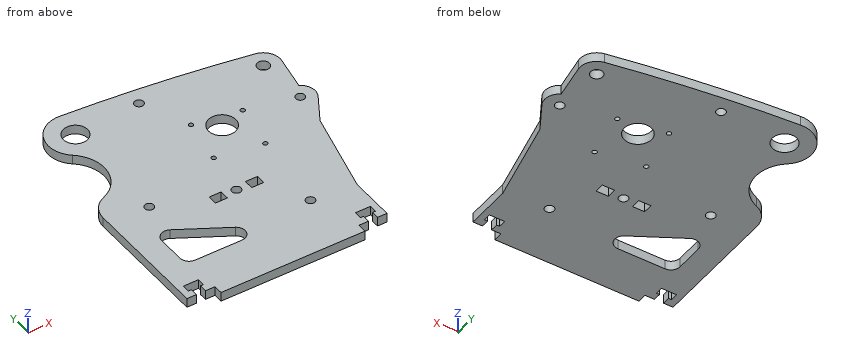
from build123d import *

# Parameters (mm, degrees)
SKETCH1_R           = 4
SKETCH1_R_2         = 8
SKETCH1_R_3         = 3
SKETCH1_R_4         = 9
BOSS_EXTRUDE1_DEPTH = 6.2
CUT_EXTRUDE1_REACH  = 156.506
SKETCH2_R           = 1.5
CUT_EXTRUDE2_REACH  = 156.506
CUT_EXTRUDE3_REACH  = 156.506
SKETCH4_R           = 3
SKETCH4_W           = 8
SKETCH4_H           = 6.2


with BuildPart() as part:
    # Sketch1 → Boss-Extrude1 (new body)
    with BuildSketch(Plane.XY):
        with BuildLine():
            Line((33.65, -83.5), (47, -26.5))
            Line((47, -26.5), (57.678304402, -8.5))
            ThreePointArc((57.678304402, -8.5), (58.708572703, -0.936463864), (54, 5.071686829))
            Line((54, 5.071686829), (58, 28.071686829))
            ThreePointArc((58, 28.071686829), (56.207110337, 36.277710094), (49.152329455, 40.836584722))
            ThreePointArc((49.152329455, 40.836584722), (-10.365453902, 50.052003716), (-70.318491494, 55.789927265))
            ThreePointArc((-70.318491494, 55.789927265), (-88.125314746, 44.440216148), (-82.611172846, 24.056567409))
            ThreePointArc((-82.611172846, 24.056567409), (-74.166284142, 2.579562371), (-88.533690885, -15.480213766))
            ThreePointArc((-88.533690885, -15.480213766), (-95.663024793, -21.178356395), (-98.35, -29.900534772))
            Line((-98.35, -29.900534772), (-98.35, -113))
            Line((-98.35, -113), (-79.85, -113))
            Line((-79.85, -113), (-79.85, -119))
            Line((-79.85, -119), (15.15, -119))
            Line((15.15, -119), (15.15, -113))
            Line((15.15, -113), (33.65, -113))
            Line((33.65, -113), (33.65, -83.5))
        make_face()
        with Locations(Location((47.15, 30, 0), (0, 0, 180))):
            Circle(SKETCH1_R, mode=Mode.SUBTRACT)
        with Locations(Location((-71.5, 38, 0), (0, 0, 180))):
            Circle(SKETCH1_R_2, mode=Mode.SUBTRACT)
        with Locations(Location((-27.65, 40.9, 0), (0, 0, 180))):
            Circle(SKETCH1_R_3, mode=Mode.SUBTRACT)
        with Locations(Location((4.85, -80.4, 0), (0, 0, 180))):
            Circle(SKETCH1_R_3, mode=Mode.SUBTRACT)
        with Locations(Location((49.25, -3.5, 0), (0, 0, 180))):
            Circle(SKETCH1_R_3, mode=Mode.SUBTRACT)
        with Locations(Location((-72, -36, 0), (0, 0, 180))):
            Circle(SKETCH1_R_3, mode=Mode.SUBTRACT)
        with Locations(Location((0, 0, 0), (0, 0, 180))):
            Circle(SKETCH1_R_4, mode=Mode.SUBTRACT)
        with BuildLine():
            Line((-82.35, -64), (-82.35, -82))
            ThreePointArc((-82.35, -82), (-80.592640687, -86.242640687), (-76.35, -88))
            Line((-76.35, -88), (-45.35, -88))
            ThreePointArc((-45.35, -88), (-39.556365472, -83.560063768), (-42.337186896, -76.81126632))
            Line((-42.337186896, -76.81126632), (-73.337186896, -58.81126632))
            ThreePointArc((-73.337186896, -58.81126632), (-79.343586593, -58.800150068), (-82.35, -64))
        make_face(mode=Mode.SUBTRACT)
    extrude(amount=BOSS_EXTRUDE1_DEPTH)

    # Sketch2 → Cut-Extrude1 (cut, up to next)
    with BuildSketch(Plane.XY.offset(6.2), mode=Mode.PRIVATE) as cut_extrude1_sk1:
        with Locations((-19.348702159, -20.792251556)):
            Circle(SKETCH2_R)
    cut_extrude1_tool1 = extrude(cut_extrude1_sk1.sketch, amount=-CUT_EXTRUDE1_REACH, mode=Mode.PRIVATE) & part.part
    # Sketch2 → Cut-Extrude1 (cut, up to next)
    with BuildSketch(Plane.XY.offset(6.2), mode=Mode.PRIVATE) as cut_extrude1_sk2:
        with Locations((11.192862241, -26.103827973)):
            Circle(SKETCH2_R)
    cut_extrude1_tool2 = extrude(cut_extrude1_sk2.sketch, amount=-CUT_EXTRUDE1_REACH, mode=Mode.PRIVATE) & part.part
    # Sketch2 → Cut-Extrude1 (cut, up to next)
    with BuildSketch(Plane.XY.offset(6.2), mode=Mode.PRIVATE) as cut_extrude1_sk3:
        with Locations((-14.037125741, 9.749312843)):
            Circle(SKETCH2_R)
    cut_extrude1_tool3 = extrude(cut_extrude1_sk3.sketch, amount=-CUT_EXTRUDE1_REACH, mode=Mode.PRIVATE) & part.part
    # Sketch2 → Cut-Extrude1 (cut, up to next)
    with BuildSketch(Plane.XY.offset(6.2), mode=Mode.PRIVATE) as cut_extrude1_sk4:
        with Locations((16.504438658, 4.437736426)):
            Circle(SKETCH2_R)
    cut_extrude1_tool4 = extrude(cut_extrude1_sk4.sketch, amount=-CUT_EXTRUDE1_REACH, mode=Mode.PRIVATE) & part.part
    add(cut_extrude1_tool1.solids().sort_by_distance((-19.348702, -20.792252, 6.2))[0], mode=Mode.SUBTRACT)
    add(cut_extrude1_tool2.solids().sort_by_distance((11.192862, -26.103828, 6.2))[0], mode=Mode.SUBTRACT)
    add(cut_extrude1_tool3.solids().sort_by_distance((-14.037126, 9.749313, 6.2))[0], mode=Mode.SUBTRACT)
    add(cut_extrude1_tool4.solids().sort_by_distance((16.504439, 4.437736, 6.2))[0], mode=Mode.SUBTRACT)

    # Sketch3 → Cut-Extrude2 (cut, up to next)
    with BuildSketch(Plane(origin=(0, 0, 0), x_dir=(-1, 0, 0), z_dir=(0, 0, -1)), mode=Mode.PRIVATE) as cut_extrude2_sk1:
        Polygon((-29.4, -103), (-19.4, -103), (-19.4, -108), (-21.4, -108), (-21.4, -113), (-27.4, -113), (-27.4, -108), (-29.4, -108), align=None)
    cut_extrude2_tool1 = extrude(cut_extrude2_sk1.sketch, amount=-CUT_EXTRUDE2_REACH, mode=Mode.PRIVATE) & part.part
    # Sketch3 → Cut-Extrude2 (cut, up to next)
    with BuildSketch(Plane(origin=(0, 0, 0), x_dir=(-1, 0, 0), z_dir=(0, 0, -1)), mode=Mode.PRIVATE) as cut_extrude2_sk2:
        Polygon((92.1, -113), (86.1, -113), (86.1, -108), (84.1, -108), (84.1, -103), (94.1, -103), (94.1, -108), (92.1, -108), align=None)
    cut_extrude2_tool2 = extrude(cut_extrude2_sk2.sketch, amount=-CUT_EXTRUDE2_REACH, mode=Mode.PRIVATE) & part.part
    add(cut_extrude2_tool1.solids().sort_by_distance((24.4, -107.375, 0))[0], mode=Mode.SUBTRACT)
    add(cut_extrude2_tool2.solids().sort_by_distance((-89.1, -107.375, 0))[0], mode=Mode.SUBTRACT)

    # Sketch4 → Cut-Extrude3 (cut, up to next)
    with BuildSketch(Plane.XY.offset(6.2), mode=Mode.PRIVATE) as cut_extrude3_sk1:
        with Locations((-24.05, -50.4)):
            Circle(SKETCH4_R)
    cut_extrude3_tool1 = extrude(cut_extrude3_sk1.sketch, amount=-CUT_EXTRUDE3_REACH, mode=Mode.PRIVATE) & part.part
    # Sketch4 → Cut-Extrude3 (cut, up to next)
    with BuildSketch(Plane.XY.offset(6.2), mode=Mode.PRIVATE) as cut_extrude3_sk2:
        with Locations((-36.05, -50.4)):
            Rectangle(SKETCH4_W, SKETCH4_H)
    cut_extrude3_tool2 = extrude(cut_extrude3_sk2.sketch, amount=-CUT_EXTRUDE3_REACH, mode=Mode.PRIVATE) & part.part
    # Sketch4 → Cut-Extrude3 (cut, up to next)
    with BuildSketch(Plane.XY.offset(6.2), mode=Mode.PRIVATE) as cut_extrude3_sk3:
        with Locations((-12.05, -50.4)):
            Rectangle(SKETCH4_W, SKETCH4_H)
    cut_extrude3_tool3 = extrude(cut_extrude3_sk3.sketch, amount=-CUT_EXTRUDE3_REACH, mode=Mode.PRIVATE) & part.part
    add(cut_extrude3_tool1.solids().sort_by_distance((-24.05, -50.4, 6.2))[0], mode=Mode.SUBTRACT)
    add(cut_extrude3_tool2.solids().sort_by_distance((-36.05, -50.4, 6.2))[0], mode=Mode.SUBTRACT)
    add(cut_extrude3_tool3.solids().sort_by_distance((-12.05, -50.4, 6.2))[0], mode=Mode.SUBTRACT)


solid = part.part
Check sheet for the modelled part. Datum: model origin and axes. Units: mm. Give positions to 0.01 mm unless a question says otherwise; leave off trailing zeros. Order: outer loops, then holes, each group sorted by start corner. A loop starts at its lowest first (then second) coordinate and runs counter-clockwise, first axis right, second up. Notation, with made-up numbers: M 84,67 L 139,67 A27 ccw 139,87 Z; hole C 81,20.5 d6. An arc over 180 degrees is marked long. Answer as CSV lines item,"result". Start each with the question number.
Item 1: Cross-section at D-D on x = 38. Enter the section's corners in (y, z), plus the area to 3 significant figures.
Item 2: Cross-section at C-C on z = 1. State how many separate pieces and enclosed holes the cut face has, plus the area to 3 significant figures.
Item 3: Gauge pin test, flat ends, axial feed: P1, Ø2, axis at x = -85, z = 4, coming from the +Y side; P2, Ø1, axis at x = -75, z = 3, coming from the +Y side; P3, Ø3, axis at y = -116, z = 3, coming from the +X side. Record the tip position at first contact, or that the pin passes through.
Item 4: Cross-section at A-A on y = -105.5. Enter the section's corners in (x, z).
Item 5: Cross-section at B-B on x = -55.5. Enter the section's corners in (y, z).
Item 6: Thickness scan on line 1 (X direction, y = -103.5, z = 5.5); line 2 (Y direction, x = -14, z = 2.5); line 3 (Y direction, x = -71.5, z = 2). Record the ranges inside material, lowest first. Write a range as [from, to].
Established:
1,outline,"M -64.93,0 L 42.83,0 L 42.83,6.2 L -64.93,6.2 Z"
1,area,"668 mm^2"
2,separate pieces,"1"
2,enclosed holes,"15"
2,area,"21,100 mm^2"
3,P1,"stops at y = 50.71"
3,P2,"stops at y = 55.57"
3,P3,"stops at x = 15.15"
4,outline,"M -98.35,0 L -94.1,0 L -94.1,6.2 L -98.35,6.2 Z; M -84.1,0 L 19.4,0 L 19.4,6.2 L -84.1,6.2 Z; M 29.4,0 L 33.65,0 L 33.65,6.2 L 29.4,6.2 Z"
5,outline,"M -119,0 L -88,0 L -88,6.2 L -119,6.2 Z; M -69.17,0 L 54.7,0 L 54.7,6.2 L -69.17,6.2 Z"
6,line 1,"x = [-98.35, -94.1], [-84.1, 19.4], [29.4, 33.65]"
6,line 2,"y = [-119, -53.5], [-47.3, 8.25], [11.25, 50.5]"
6,line 3,"y = [-119, -88], [-59.88, -38.96], [-33.04, 30], [46, 55.83]"
